The listing builds one solid part. Answer for the finished solid, in the listing's coordinates (mm). A direction names the side the tool comes from. Coordinates: 2 decimals unless noted, no trailing zeros. Order: outer loops, then holes, each group sorted by start corner. A loop starts at its lowest first (then second) coordinate and runs counter-clockwise, first axis right, second up. Notation, with made-up numbers: (59, 42) -> (80, 42) arc R24 ccw to (80, 63) -> close; hole circle Ø1 at (32.5, 74.25). An arc over 180 degrees is marked (long way). Write each question's results on one line, items separated by ' | '. Start each with the question number.
(1) A tool of negligible diameter and unlimited length cuts with its end or side. For faces 5 (the face through (2, 3, 0)), 6 (the face through (1.75, 1.711, -24.696)), from which of +Z, -Z, +X, -X, +Y, -Y can it reach the whole face along a straight path? Write none if from no direction.
(2) The part is cut by section C-C, the plane z = 17.5. Give the vertices of the cut face in (x, y).
(3) Straight lines are drawn through the part: L1, parallel to Z at x = -97, y = 15; L2, parallel to Y at x = -112.5, z = 11.5; L3, parallel to Y at x = -2, z = -24. For each, find the intervals that lie inside material, in ascending order.
(4) Determine the mould class of faces 1 (the face through (2, 22, 23.5)), 2 (the face through (1.75, 1.804, 24.789)), 3 (the face through (2, 22, -23.5)), 4 (the face through (2, 0, 0)) for opening direction Z: +Z half, -Z half, draft (parallel to the pull), parting line (faces both ways), or undercut.
(5) Given pin 1 (1.5 mm diameter, centred on x = 38.5, z = -6.5, fed in from +Y), flat-ended and moving along its own axis, determine where the tip first touches the part or whether it passes through.
(6) The part is cut by section B-B, the plane x = -64. Give the vertices of the cut face in (y, z).
(7) The part is cut by section A-A, the plane y = 31. Give the vertices of the cut face in (x, z).
```python
from build123d import *

# Parameters (mm, degrees)
TRACK_DEPTH = 125


with BuildPart() as part:
    # 草图1 → Track (new, symmetric)
    with BuildSketch(Plane(origin=(0, 0, 0), x_dir=(0, 0, -1), z_dir=(1, 0, 0))):
        with BuildLine():
            Line((-26.5, 38.5), (-26.5, 6))
            ThreePointArc((-26.5, 6), (-24.742640687, 1.757359313), (-20.5, 0))
            Line((-20.5, 0), (20.5, 0))
            ThreePointArc((20.5, 0), (24.742640687, 1.757359313), (26.5, 6))
            Line((26.5, 6), (26.5, 38.5))
            Line((26.5, 38.5), (23.5, 38.5))
            Line((23.5, 38.5), (23.5, 6))
            ThreePointArc((23.5, 6), (22.621320344, 3.878679656), (20.5, 3))
            Line((20.5, 3), (-20.5, 3))
            ThreePointArc((-20.5, 3), (-22.621320344, 3.878679656), (-23.5, 6))
            Line((-23.5, 6), (-23.5, 38.5))
            Line((-23.5, 38.5), (-26.5, 38.5))
        make_face()
    extrude(amount=TRACK_DEPTH, both=True)


solid = part.part
```
Established:
1) face 5: +X, -X, +Y | face 6: -Z, +X, -X, -Y
2) outline: (-125, 0) -> (125, 0) -> (125, 3) -> (-125, 3) -> close
3) L1: z = -26.5 to -23.5, 23.5 to 26.5 | L2: y = 0 to 3 | L3: y = 1.13 to 38.5
4) face 1: undercut | face 2: +Z half | face 3: undercut | face 4: draft
5) pin 1: stops at y = 3
6) outline: (0, -20.5) arc R6 ccw to (6, -26.5) -> (38.5, -26.5) -> (38.5, -23.5) -> (6, -23.5) arc R3 cw to (3, -20.5) -> (3, 20.5) arc R3 cw to (6, 23.5) -> (38.5, 23.5) -> (38.5, 26.5) -> (6, 26.5) arc R6 ccw to (0, 20.5) -> close
7) outline: (-125, -26.5) -> (125, -26.5) -> (125, -23.5) -> (-125, -23.5) -> close; (-125, 23.5) -> (125, 23.5) -> (125, 26.5) -> (-125, 26.5) -> close
